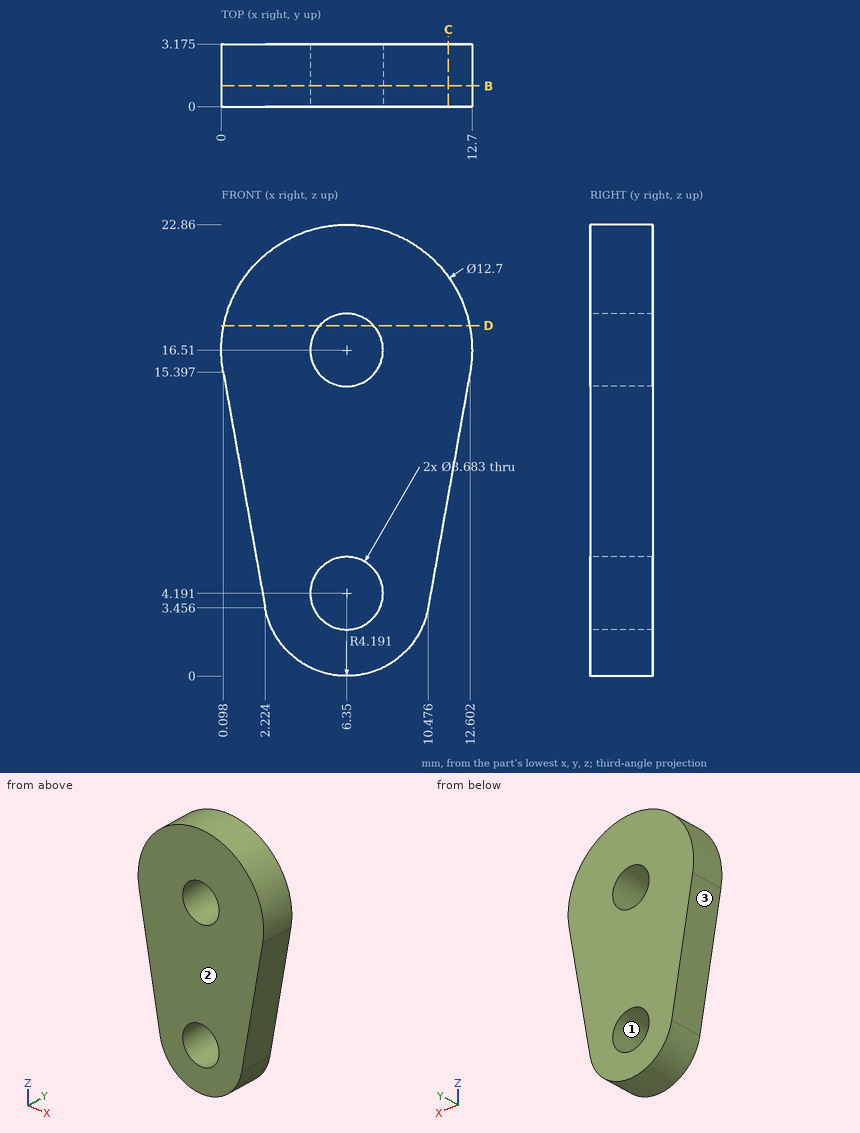
Study the drawing (mm; zero at the part's minimum x, y, z) and answer. Round coordinates to 2 decimals unless told otherwise and drop trailing zeros. Loops run counter-clockwise (first coordinate to the right, second up) from the corner with the lowest first, then second, coordinate; pieces in that order, holes last. Notation, with made-up numbers: (41, -31.75) -> (99, -31.75) arc R6 ccw to (99, -21.75) -> close; hole circle Ø5 at (39, -15). An arc over 180 degrees is marked (long way). One line per item, written item: value.
1) A cutting plane is placed at D-D (z = 17.75). Determine the outline of the cut face in (x, y) (1 decimal).
Answer list:
outline: (0.1, 0) -> (5, 0) -> (5, 3.2) -> (0.1, 3.2) -> close; (7.7, 0) -> (12.6, 0) -> (12.6, 3.2) -> (7.7, 3.2) -> close
2) A cutting plane is placed at B-B (y = 1.05). Determine the outline of the cut face in (x, z).
Answer list:
outline: (0.1, 15.4) -> (2.22, 3.46) arc R4.19 ccw to (10.48, 3.46) -> (12.6, 15.4) arc R6.35 ccw (long way) to start; hole circle Ø3.68 at (6.35, 4.19); hole circle Ø3.68 at (6.35, 16.51)
3) The mould has two halves that part along Z. Classify the marked faces 1, 2 and 3: pulls with the +Z half, pulls with the -Z half, needs draft (parallel to the pull), parting line crosses it, or undercut.
Answer list:
face 1: undercut
face 2: needs draft
face 3: pulls with the -Z half
4) Consider L1, parallel to Z at x = 6.25, y = 1.85; L2, parallel to X at y = 2.45, z = 16.5; L3, parallel to Z at x = 5.5, y = 1.6 (1 decimal). Determine where each line is inside the solid, lowest interval first. Write a range as [from, to].
Answer list:
L1: z = [0, 2.35], [6.03, 14.67], [18.35, 22.86]
L2: x = [0, 4.51], [8.19, 12.7]
L3: z = [0.1, 2.6], [5.8, 14.9], [18.1, 22.8]
5) A cutting plane is placed at C-C (x = 11.5). Determine the outline of the cut face in (y, z) (1 decimal).
Answer list:
outline: (0, 9.2) -> (3.2, 9.2) -> (3.2, 20.2) -> (0, 20.2) -> close
